Source: CAD feature listing. Evaluate the final solid. Frame: model axes, mm. Give positions to 0.01 mm unless a question says otherwise; leave off trailing zeros. Order: outer loops, then holes, each group sorted by start corner. A loop starts at its lowest first (then second) coordinate and runs counter-clockwise, first axis right, second up. Notation, with made-up numbers: M 25,51 L 56,51 A14 ccw 56,58 Z; hole C 51.5,50.5 d5. An arc over 180 degrees is marked long. Use CSV: the item, a comma, the result in double quotes. Start each with the question number.
1. Mould query, pull axis X, two halves, no side actions, for faces 1 (the cylindrical face through (-122.5, 25.6, 2.9)), 2 (the flat face through (41.401, 49.3, 69.643)), 3 (the flat face through (-41.401, 49.3, -69.643)), 4 (the cylindrical face through (122.5, 25.6, 2.9)). Classes: released by +X, released by -X, zero draft, split by the parting line, or undercut.
2. Line query: line 1 along Z through (x, y) = (-10.5, 87); line 2 along X through (y, z) = (53, -26); line 3 along X through (y, z) = (35.5, 29.5). Output: solid intervals per line, ascending. Write a range as [from, to].
3. Section query A-A, the plane y = 15. Return the cut outline in (x, z).
4. Pin query (flat end, axial travel): P1, Ø4, axis at x = -35.5, y = 88, coming from the -Z side; P2, Ø3, axis at y = 43.5, z = -38, coming from the -X side; P3, Ø10, axis at x = -100, z = 12, coming from the +Y side. Return the tip coordinate at first contact, or that it passes through.
5. Section query B-B, the plane x = 17.5. Return the cut outline in (y, z), plus the area to 3 significant figures.
6. Section query C-C, the plane y = 61.5. Return the cut outline in (x, z), plus the area to 3 significant figures.
7. Section query D-D, the plane x = 66. Return the cut outline in (y, z), plus the area to 3 significant figures.
from build123d import *

# Parameters (mm, degrees)
BOSS_EXTRUDE1_DEPTH = 100
SKETCH6_R           = 32.5
CUT_EXTRUDE1_DEPTH  = 160.58632929
SKETCH7_R           = 25
BOSS_EXTRUDE2_DEPTH = 84


with BuildPart() as part:
    # Sketch5 → Boss-Extrude1 (new body)
    with BuildSketch(Plane(origin=(0, 0, 0), x_dir=(1, 0, 0), z_dir=(0, 1, 0))):
        Polygon((-80.025635128, -48.453021269), (1.948729745, -93.530743609), (81.974364872, -45.07772234), (80.025635128, 48.453021269), (-1.948729745, 93.530743609), (-81.974364872, 45.07772234), align=None)
    extrude(amount=BOSS_EXTRUDE1_DEPTH)

    # Sketch6 → Cut-Extrude1 (cut, through all)
    with BuildSketch(Plane(origin=(0, 0, 0), x_dir=(-1, 0, 0), z_dir=(0, -1, 0))):
        with Locations(Location((0, 0, 0), (0, 0, 90))):
            Circle(SKETCH6_R)
    extrude(amount=-CUT_EXTRUDE1_DEPTH, mode=Mode.SUBTRACT)

    # Sketch7 → Boss-Extrude2 (add)
    with BuildSketch(Plane(origin=(81, 0, -1.687649464), x_dir=(-0.020830657718770396, 0, -0.9997830183089746), z_dir=(0.9997830183089746, 0, -0.020830657718770396))):
        with Locations((0, 50)):
            Circle(SKETCH7_R)
    boss_extrude2 = extrude(amount=BOSS_EXTRUDE2_DEPTH)

    # Mirror1: Boss-Extrude2 across plane
    add(boss_extrude2.mirror(Plane(origin=(0, 0, 0), x_dir=(0, 0, 1), z_dir=(1, 0, 0))))


solid = part.part
Result set:
1,face 1,"undercut"
1,face 2,"released by +X"
1,face 3,"released by -X"
1,face 4,"undercut"
2,line 1,"[-88.35, -30.76], [30.76, 86.69]"
2,line 2,"[-164.51, -19.5], [19.5, 164.51]"
2,line 3,"[-80.42, -13.64], [13.64, 81.65]"
3,outline,"M -81.97,-45.08 L -1.95,-93.53 L 80.03,-48.45 L 81.97,45.08 L 1.95,93.53 L -80.03,48.45 Z; hole C 0,0 d65"
4,P1,"z = -74.43"
4,P2,"x = -81.86"
4,P3,"y = 73.29"
5,outline,"M 0,-82.84 L 100,-82.84 L 100,-27.39 L 0,-27.39 Z; M 0,27.39 L 100,27.39 L 100,84.11 L 0,84.11 Z"
5,area,"11,200 mm2"
6,outline,"M -165.44,18.76 L -164.52,-25.63 L -81.53,-23.9 L -81.97,-45.08 L -1.95,-93.53 L 80.03,-48.45 L 80.54,-23.88 L 164.52,-25.63 L 165.44,18.76 L 81.46,20.51 L 81.97,45.08 L 1.95,93.53 L -80.03,48.45 L -81.04,0 L -81.46,20.51 Z; hole C 0,0 d65"
6,area,"26,900 mm2"
7,outline,"M 0,-56.17 L 100,-56.17 L 100,54.75 L 0,54.75 Z"
7,area,"11,100 mm2"
